Check sheet for the drawn part. Datum: minimum x, y, z corner. Units: mm. Round coordinates to 2 decimals unless told otherwise and drop trailing zeros. Write each loop counter-clockwise with the first axis right and the second up, starting at its lowest first coordinate (ties: lowest second). Pieces come first, ordered by that corner, then holes. Notation, with made-up numbers: M -12,-8.5 L 24,-8.5 A35 cw 24,27.5 Z; hole C 7,31.5 d9. An arc over 180 degrees is marked long. One line per item, written item: value. Start each with the question number.
Item 1: Section check D-D, the plane y = 13.5. Record the cut outline in (x, z), then the cut area to 3 significant figures.
Item 2: Gauge pin test, flat ends, axial feed: pin 1 (4.5 mm diameter, centred on x = 6.5, z = 6, fed in from +Y); pin 2 (5 mm diameter, centred on x = 6.5, y = 31, fed in from +Z); pin 3 (4 mm diameter, centred on y = 29, z = 6, fed in from -X); pin 4 (1 mm diameter, centred on y = 22, z = 4.5, fed in from +X). Record the tip position at first contact, or that the pin passes through.
Item 3: Thickness scan on probe 1 along Y at (x, z) = (5, 1.5); probe 2 along X at (y, z) = (26.5, 5.25); probe 3 along Z at (x, y) = (5.75, 19). Record the ranges inside material, lowest first. Write a range as from..to.
Item 4: Draft check along Y on the marked faces 1, 2 and 3. Enter one of: +Y half, -Y half, draft (parallel to the pull), parting line (faces both ways), or undercut.
Item 5: Section check C-C, the plane y = 37. Record the cut outline in (x, z).
Item 6: Section check B-B, the plane x = 5. Record the cut outline in (y, z).
Item 7: Section check A-A, the plane z = 5. Record the cut outline in (x, y), then the cut area to 3 significant figures.
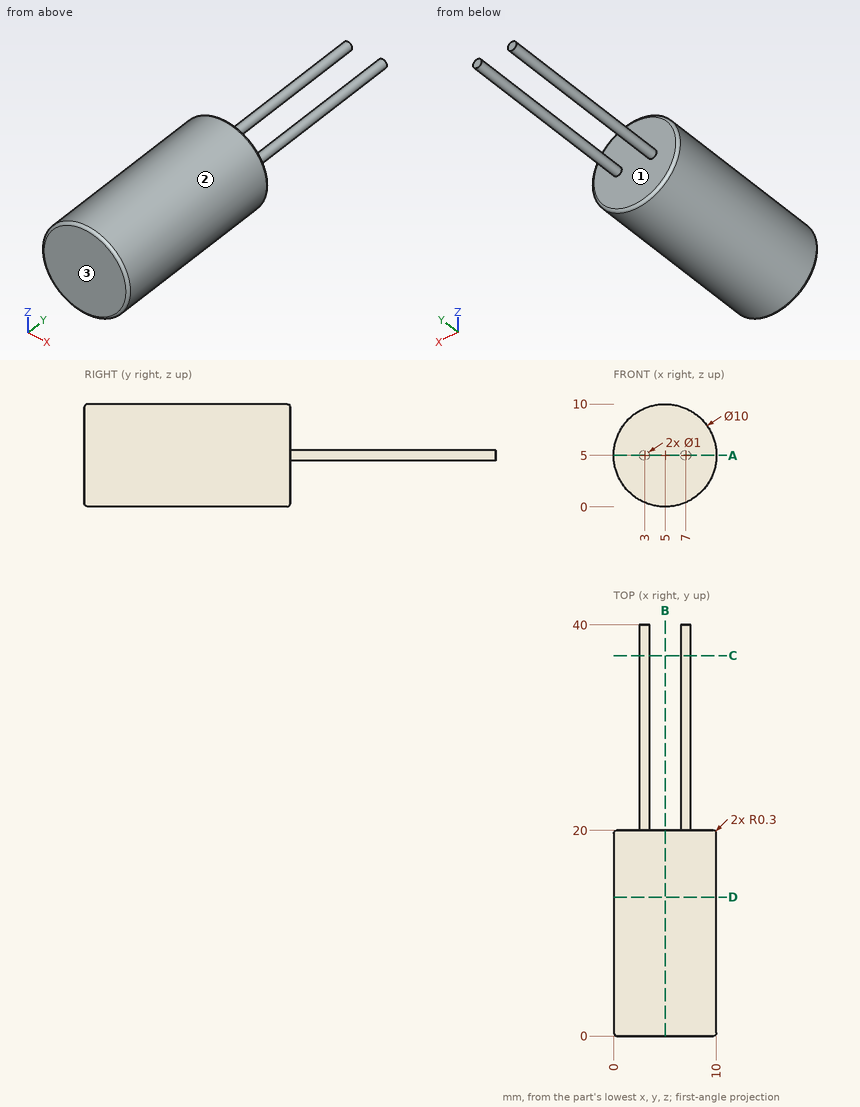
Response values:
1. outline: C 5,5 d10
1. area: 78.5 mm2
2. pin 1: stops at y = 40
2. pin 2: stops at z = 5.5
2. pin 3: stops at x = 2.5
2. pin 4: stops at x = 7.5
3. probe 1: y = 0..20
3. probe 2: x = 2.57..3.43, 6.57..7.43
3. probe 3: z = 0.06..9.94
4. face 1: +Y half
4. face 2: draft
4. face 3: -Y half
5. outline: C 3,5 d1; C 7,5 d1
6. outline: M 0,0.3 A0.3 ccw 0.3,0 L 19.7,0 A0.3 ccw 20,0.3 L 20,9.7 A0.3 ccw 19.7,10 L 0.3,10 A0.3 ccw 0,9.7 Z
7. outline: M 0,0.3 A0.3 ccw 0.3,0 L 9.7,0 A0.3 ccw 10,0.3 L 10,19.7 A0.3 ccw 9.7,20 L 7.5,20 L 7.5,40 L 6.5,40 L 6.5,20 L 3.5,20 L 3.5,40 L 2.5,40 L 2.5,20 L 0.3,20 A0.3 ccw 0,19.7 Z
7. area: 240 mm2
